Geometry check sheet. Reference: the model listing, model coordinates, mm. A direction names the side the tool comes from. Give positions to 0.01 mm unless a question says otherwise; leave off trailing zeros. Loops run counter-clockwise (first coordinate to the right, second up) from the corner with the lowest first, then second, coordinate; pieces in that order, holes last. Notation, with made-up numbers: (0.5, -2) -> (42.5, -2) arc R18 ccw to (42.5, 26) -> close; hole circle Ø4 at (37.25, 54.5). An arc over 180 degrees is marked (long way). Answer as a JSON object with one key per item and string values.
from build123d import *

# Parameters (mm, degrees)
BOSS_EXTRUDE1_DEPTH                            = 138.88615
SKETCH3_R                                      = 2
CUT_EXTRUDE2_DEPTH                             = 100
LPATTERN1_COUNT                                = 16
LPATTERN1_PITCH                                = 8
FILLET1_R                                      = 1
CSK_FOR_M4_FLAT_HEAD_MACHINE_SCREW1_AT_2_COUNT = 2
CSK_FOR_M4_FLAT_HEAD_MACHINE_SCREW1_AT_2_PITCH = 118.88615
CSK_FOR_M4_FLAT_HEAD_MACHINE_SCREW1_AT_3_COUNT = 2
CSK_FOR_M4_FLAT_HEAD_MACHINE_SCREW1_AT_3_PITCH = 101.76615


with BuildPart() as part:
    # Sketch1 → Boss-Extrude1 (new body)
    with BuildSketch(Plane.XY):
        Polygon((-9, 0), (9, 0), (11.309401077, 4), (9, 8), (12.5, 8), (12.5, -3), (-12.5, -3), (-12.5, 8), (-9, 8), (-11.309401077, 4), align=None)
    extrude(amount=-BOSS_EXTRUDE1_DEPTH)

    # Sketch3 → Cut-Extrude2 (cut)
    with BuildSketch(Plane(origin=(12.5, 0, 0), x_dir=(0, 0, -1), z_dir=(1, 0, 0))):
        with Locations((8, 4)):
            Circle(SKETCH3_R)
    cut_extrude2 = extrude(amount=-CUT_EXTRUDE2_DEPTH, mode=Mode.SUBTRACT)

    # LPattern1: Cut-Extrude2 ×16
    with Locations(*[(0, 0, -i * LPATTERN1_PITCH) for i in range(1, LPATTERN1_COUNT)]):
        add(cut_extrude2, mode=Mode.SUBTRACT)

    # Fillet1
    fillet1_edges = [part.edges().sort_by_distance(p)[0] for p in [
        (12.5, -3, -69.443075),
        (-12.5, -3, -69.443075),
    ]]
    fillet(fillet1_edges, radius=FILLET1_R)

    # Sketch5 → CSK for M4 Flat Head Machine Screw1 (revolve, cut)
    with BuildSketch(Plane(origin=(0, 0, -10), x_dir=(0, 0, 1), z_dir=(1, 0, 0))):
        Polygon((0, 0), (0, 3), (2.25, 3), (2.25, 2.45), (4.7, 0), align=None)
    csk_for_m4_flat_head_machine_screw1 = revolve(axis=Axis((0, 6.35, -10), (0, -1, 0)), mode=Mode.SUBTRACT)

    # CSK for M4 Flat Head Machine Screw1 at 2: CSK for M4 Flat Head Machine Screw1 ×2
    with Locations(*[(0, 0, -i * CSK_FOR_M4_FLAT_HEAD_MACHINE_SCREW1_AT_2_PITCH) for i in range(1, CSK_FOR_M4_FLAT_HEAD_MACHINE_SCREW1_AT_2_COUNT)]):
        add(csk_for_m4_flat_head_machine_screw1, mode=Mode.SUBTRACT)

    # CSK for M4 Flat Head Machine Screw1 at 3: CSK for M4 Flat Head Machine Screw1 ×2
    with Locations(*[(0, 0, -i * CSK_FOR_M4_FLAT_HEAD_MACHINE_SCREW1_AT_3_PITCH) for i in range(1, CSK_FOR_M4_FLAT_HEAD_MACHINE_SCREW1_AT_3_COUNT)]):
        add(csk_for_m4_flat_head_machine_screw1, mode=Mode.SUBTRACT)


solid = part.part
1) Draft check along X on faces 1 (the face through (12.5, 3, -68)), 2 (the face through (-10.17, 2.03, -68.47)). Enter one of: pulls with the +X half, pulls with the -X half, needs draft (parallel to the pull), parting line crosses it, or undercut.
Geometry check:
{"face 1": "pulls with the +X half", "face 2": "undercut"}
2) Depth check by flat-ended pin: P1, Ø3.5, axis at y = 4, z = -120, coming from the +X side. Enter the tip coordinate at first touch or a pass-through.
Geometry check:
{"P1": "passes through"}
3) Section check B-B on x = 6.75. Record the cut outline in (y, z), plus the area to 3 significant figures.
Geometry check:
{"outline": "(-3, -138.89) -> (0, -138.89) -> (0, 0) -> (-3, 0) -> close", "area": "417 mm2"}
4) Material ranges on line 1 along Y through (x, z) = (-10.75, -128); line 2 along X through (y, z) = (6, -78.5); line 3 along Y through (x, z) = (4, -100), recorded low to high. Write a range as from..to.
Geometry check:
{"line 1": "y = -3..2, 6..8", "line 2": "x = -12.5..-10.15, 10.15..12.5", "line 3": "y = -3..0"}
5) Section check A-A on z = -16.5. Record the cut outline in (x, y).
Geometry check:
{"outline": "(-12.5, -2) arc R1 ccw to (-11.5, -3) -> (11.5, -3) arc R1 ccw to (12.5, -2) -> (12.5, 2.06) -> (10.19, 2.06) -> (9, 0) -> (-9, 0) -> (-10.19, 2.06) -> (-12.5, 2.06) -> close; (-12.5, 5.94) -> (-10.19, 5.94) -> (-9, 8) -> (-12.5, 8) -> close; (9, 8) -> (10.19, 5.94) -> (12.5, 5.94) -> (12.5, 8) -> close"}
6) Tool access check on faces 3 (the face through (-11.564, 4.601, -81.908)), 4 (the face through (10.17, 5.97, -68.47)). Record the directions out of +Z, -Z, +X, -X, +Y, -Y that give a thin tool (end or side, any length) a straight path to the whole face; none if there is none.
Geometry check:
{"face 3": "+X, -X", "face 4": "+Z, -Z"}
7) Section check C-C on z = -80. Record the cut outline in (x, y).
Geometry check:
{"outline": "(-12.5, -2) arc R1 ccw to (-11.5, -3) -> (11.5, -3) arc R1 ccw to (12.5, -2) -> (12.5, 2) -> (10.15, 2) -> (9, 0) -> (-9, 0) -> (-10.15, 2) -> (-12.5, 2) -> close; (-12.5, 6) -> (-10.15, 6) -> (-9, 8) -> (-12.5, 8) -> close; (9, 8) -> (10.15, 6) -> (12.5, 6) -> (12.5, 8) -> close"}
